Could you check a few things on this drawing? It's one solid part, dimensions in mm from its lowest x, y, z. Round coordinates to 2 decimals unless told otherwise and drop trailing zeros. Write each loop counter-clockwise with the first axis right and the second up, starting at its lowest first coordinate (ties: lowest second). Pieces come first, ordered by that corner, then holes. Notation, with made-up numbers: (66, -2.5) - (107, -2.5) arc R29 ccw to (107, 18.5) - close; hole circle Ø11 at (-24.5, -9.5). An arc over 180 degrees is marked (long way). Use one line per item in the form item = value. Start each with the question number.
1. I want a section at B-B, the plane z = 352.5. List the corners of the cut face in (x, y) for me, plus the area to 3 significant figures.
2. We'd pull the mould along X, two halves only. Please class the marked faces 1, 2, 3 and 4: +X half, -X half, draft (parallel to the pull), parting line (faces both ways), or undercut.
3. I want a section at A-A, the plane y = 90. List the corners of the cut face in (x, z) for me.
4. Will this pin go through, and if not, where does the flat tip stop? pin 1 (2 mm diameter, centred on x = 906.5, z = 472.5, fed in from -Y).
5. I want a section at C-C, the plane x = 846. List the corners of the cut face in (y, z) for me.
6. If I drill on line 1 along X through (y, z) = (121, 650); line 2 along X through (y, z) = (331, 558); line 3 along Y through (x, z) = (481, 371.5), over which ranges is the centre line in solid material (lowest first)?
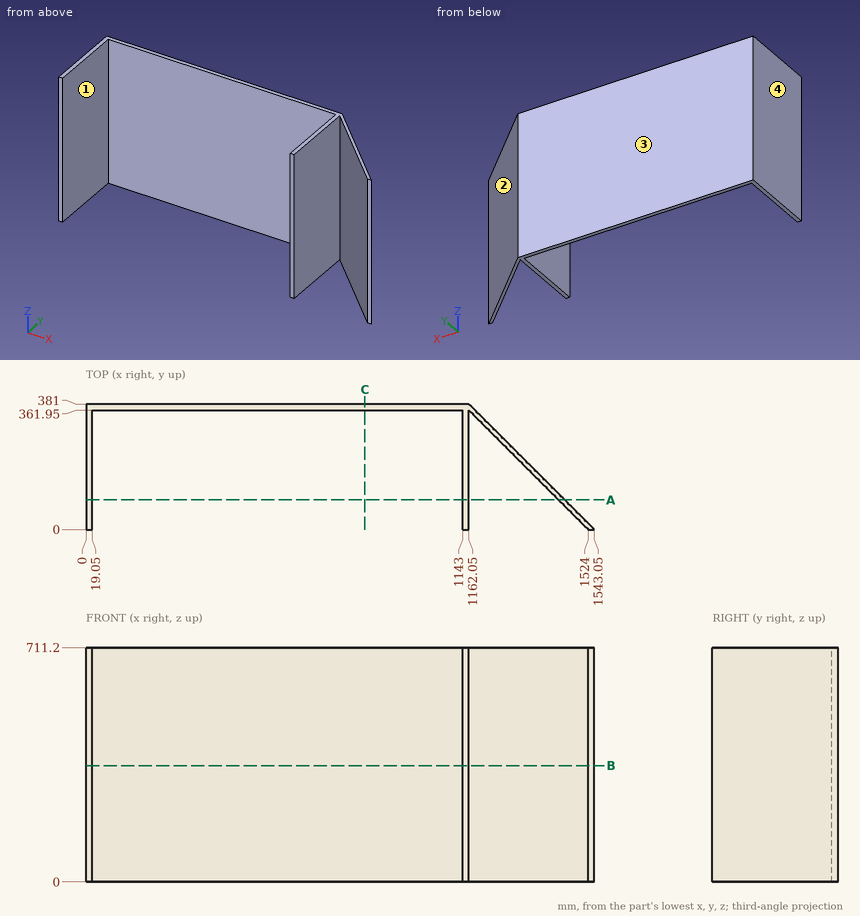
Model answer:
q1.outline = (0, 0) - (19.05, 0) - (19.05, 361.95) - (1143, 361.95) - (1143, 0) - (1162.05, 0) - (1162.05, 361.95) - (1524, 0) - (1543.05, 0) - (1162.05, 381) - (0, 381) - close
q1.area = 43,000 mm2
q2.face_1 = undercut
q2.face_2 = +X half
q2.face_3 = draft
q2.face_4 = -X half
q3.outline = (0, 0) - (19.05, 0) - (19.05, 711.2) - (0, 711.2) - close; (1143, 0) - (1162.05, 0) - (1162.05, 711.2) - (1143, 711.2) - close; (1434, 0) - (1453.05, 0) - (1453.05, 711.2) - (1434, 711.2) - close
q4.pin_1 = 361.95
q5.outline = (361.95, 0) - (381, 0) - (381, 711.2) - (361.95, 711.2) - close
q6.line_1 = 0 to 19.05, 1143 to 1162.05, 1403 to 1422.05
q6.line_2 = 0 to 19.05, 1143 to 1162.05, 1193 to 1212.05
q6.line_3 = 361.95 to 381
